Autodesk Inventor part; units mm, degrees
ref_plane "YZ Plane" through (0, 0, 0) normal (1, 0, 0) x (0, 1, 0)
ref_plane "XZ Plane" through (0, 0, 0) normal (0, 1, 0) x (-1, 0, 0)
ref_plane "XY Plane" through (0, 0, 0) normal (0, 0, 1) x (1, 0, 0)
sketch "Sketch2" plane through (0, 0, 0) normal (0, 1, 0) x (-1, 0, 0)
  line L0 (0, 0) -> (-59, 0)
  line L1 (-59, 0) -> (-59, 78)
  line L2 (-59, 78) -> (0, 78)
  line L3 (0, 78) -> (0, 0)
  dimension "d0" = 59
  dimension "d1" = 78
extrude "Extrusion1" add sketch "Sketch2" along normal blind 25
shell "Shell1" thickness 3 removed faces 1 at (39.3333, 25, 52)
sketch "Sketch4" plane through (59, 0, 0) normal (0, 0, -1) x (-1, 0, 0)
  point P0 (59, 0)
sketch "Sketch5" plane through (3, 3, 3) normal (0, 0, 1) x (1, 0, 0)
  line L0 (0, 0) -> (0, 22)
  line L1 (0, 22) -> (53, 22)
  line L2 (0, 0) -> (53, 0)
  line L3 (53, 0) -> (53, 22)
  line L4 (53, 22) -> (0, 22)
  line L5 (0, 22) -> (0, 0)
  point P0 (-3, -3)
extrude "Extrusion3" cut sketch "Sketch5" against normal blind 10
sketch "Sketch6" plane through (0, 0, 0) normal (-1, 0, 0) x (0, 0, 1)
  line L0 (4.5, 21.5) -> (30.5, 21.5)
  line L1 (30.5, 21.5) -> (30.5, 17.5)
  line L2 (30.5, 17.5) -> (4.5, 17.5)
  line L3 (4.5, 17.5) -> (4.5, 21.5)
  line L4 (0, 0) -> (0, 25)
  line L5 (0, 0) -> (78, 0)
  dimension "d19" = 26
  dimension "d20" = 4
  dimension "d21" = 4.5
  dimension "d22" = 17.5
extrude "Extrusion4" cut sketch "Sketch6" against normal through all
properties part number "arduino array box v03"
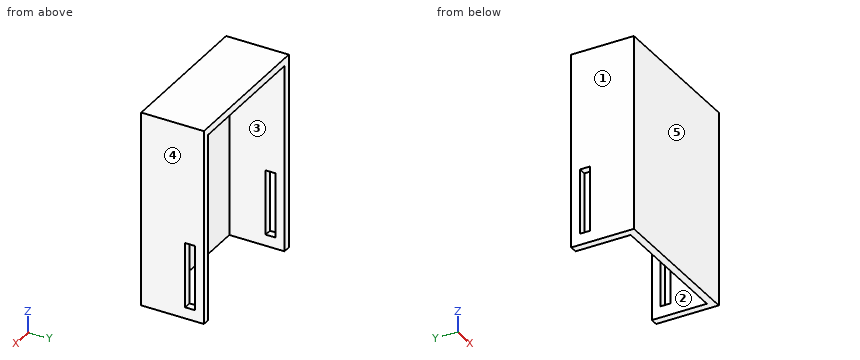
Model file for the job. Use its own axes, mm. Face numbers are marked on the shaded views. A direction names the side the tool comes from. Coordinates: 2 decimals unless noted, no trailing zeros. Order: outer loops, then holes, each group sorted by start corner. A loop starts at its lowest first (then second) coordinate and runs counter-clockwise, first axis right, second up. Notation, with made-up numbers: (37.25, -5.75) -> (95.25, -5.75) arc R22 cw to (95.25, 9.25) -> close; hole circle Ø9 at (85.25, -25). An arc over 180 degrees is marked (long way). Answer as a JSON object with one key per item and string values. Group by question number.
1) Cut at C-C, the plane y = 13. Write the cut outline in (x, z), then the cut area to 3 significant figures.
2) Cut at A-A, the plane z = 7.5. Write the cut outline in (x, y), then the cut area to 3 significant figures.
3) Which spindle directions (+Z, -Z, +X, -X, +Y, -Y) get a long thin tool onto all of the face, cutting with end or side? Do the marked faces 1 and 2. Say none if no direction does.
4) Flat gauge pins, fed straight in: pin 1 (6.5 mm diameter, centred on y = 9.5, z = 36.5, fed in from -X); pin 2 (5 mm diameter, centred on x = 49.5, y = 9, fed in from -Z); pin 3 (4 mm diameter, centred on x = 45.5, z = 62.5, fed in from +Y). Where does each tip first touch, or does it go through?
5) Cut at B-B, the plane y = 18.5. Write the cut outline in (x, z).
6) Drill centre lines: L1, parallel to X at y = 3.25, z = 33.5; L2, parallel to Y at x = 7, z = 36.5; L3, parallel to Z at x = 55, y = 19.75. Where is each one in solid material? Low to high.
7) Cut at D-D, the plane z = 46.5. Write the cut outline in (x, y), then the cut area to 3 significant figures.
8) Pull direction X, two halves, no side cores. Call the marked faces 3, 4 and 5: +X half, -X half, draft (parallel to the pull), parting line (faces both ways), or undercut.
Check values:
{
 "1": {"outline": "(0, 0) -> (3, 0) -> (3, 75) -> (56, 75) -> (56, 0) -> (59, 0) -> (59, 78) -> (0, 78) -> close", "area": "627 mm²"},
 "2": {"outline": "(0, 0) -> (59, 0) -> (59, 17.5) -> (56, 17.5) -> (56, 3) -> (3, 3) -> (3, 17.5) -> (0, 17.5) -> close; (0, 21.5) -> (3, 21.5) -> (3, 25) -> (0, 25) -> close; (56, 21.5) -> (59, 21.5) -> (59, 25) -> (56, 25) -> close", "area": "285 mm²"},
 "3": {"face 1": "+Z, -Z, -X, +Y, -Y", "face 2": "-Z, +Y"},
 "4": {"pin 1": "stops at x = 0", "pin 2": "stops at z = 75", "pin 3": "stops at y = 3"},
 "5": {"outline": "(0, 0) -> (3, 0) -> (3, 4.5) -> (0, 4.5) -> close; (0, 30.5) -> (3, 30.5) -> (3, 75) -> (56, 75) -> (56, 30.5) -> (59, 30.5) -> (59, 78) -> (0, 78) -> close; (56, 0) -> (59, 0) -> (59, 4.5) -> (56, 4.5) -> close"},
 "6": {"L1": "x = 0 to 3, 56 to 59", "L2": "y = 0 to 3", "L3": "z = 75 to 78"},
 "7": {"outline": "(0, 0) -> (59, 0) -> (59, 25) -> (56, 25) -> (56, 3) -> (3, 3) -> (3, 25) -> (0, 25) -> close", "area": "309 mm²"},
 "8": {"face 3": "undercut", "face 4": "+X half", "face 5": "draft"}
}
